Build history of the part. All positions in model axes, mm. Face numbers are marked on the shaded views. Give positions to 0.01 mm unless a question says otherwise; leave off trailing zeros. Order: outer loops, then holes, each group sorted by start corner. A loop starts at its lowest first (then second) coordinate and runs counter-clockwise, first axis right, second up. Notation, with made-up numbers: (33, -7.75) -> (44, -7.75) arc R15 cw to (44, 16.25) -> close; hole circle Ø1 at (-25.5, 61.25). An arc over 180 degrees is marked (long way). Write item = value, one per line. Start each with the question number.
from build123d import *

# Parameters (mm, degrees)
SKETCH_1_W          = 8
SKETCH_1_H          = 5
SKETCH_1_R          = 1.949999999
SKETCH_1_R_2        = 4
SKETCH_1_R_3        = 2
BOSS_EXTRUDE1_DEPTH = 10


with BuildPart() as part:
    # Sketch 1 → Boss-Extrude1 (new body)
    with BuildSketch(Plane.XY):
        with BuildLine():
            ThreePointArc((27.5, 18), (33.863961031, 15.363961031), (36.5, 9))
            Line((36.5, 9), (36.5, 41))
            Line((36.5, 41), (-6.9, 41))
            ThreePointArc((-6.9, 41), (-1.243145751, 38.656854249), (1.1, 33))
            Line((1.1, 33), (1.1, 28))
            ThreePointArc((1.1, 28), (4.028932188, 20.928932188), (11.1, 18))
            Line((11.1, 18), (27.5, 18))
        make_face()
        with BuildLine():
            ThreePointArc((-27.5, 12), (-33.5, 6), (-27.5, 0))
            Line((-27.5, 0), (27.5, 0))
            ThreePointArc((27.5, 0), (33.863961031, 2.636038969), (36.5, 9))
            ThreePointArc((36.5, 9), (33.863961031, 15.363961031), (27.5, 18))
            Line((27.5, 18), (11.1, 18))
            ThreePointArc((11.1, 18), (4.028932188, 20.928932188), (1.1, 28))
            Line((1.1, 28), (1.1, 33))
            ThreePointArc((1.1, 33), (-1.243145751, 38.656854249), (-6.9, 41))
            ThreePointArc((-6.9, 41), (-12.556854249, 38.656854249), (-14.9, 33))
            Line((-14.9, 33), (-14.9, 22))
            ThreePointArc((-14.9, 22), (-17.828932188, 14.928932188), (-24.9, 12))
            Line((-24.9, 12), (-27.5, 12))
        make_face()
        with Locations((-11.5, 6)):
            Rectangle(SKETCH_1_W, SKETCH_1_H, mode=Mode.SUBTRACT)
        with Locations((-1.238171752, 11.18329463)):
            Circle(SKETCH_1_R, mode=Mode.SUBTRACT)
        with Locations((6.5, 6)):
            Rectangle(SKETCH_1_W, SKETCH_1_H, mode=Mode.SUBTRACT)
        with Locations((27.5, 9)):
            Circle(SKETCH_1_R_2, mode=Mode.SUBTRACT)
        with Locations((-6.9, 33)):
            Circle(SKETCH_1_R_3, mode=Mode.SUBTRACT)
    extrude(amount=BOSS_EXTRUDE1_DEPTH)


solid = part.part
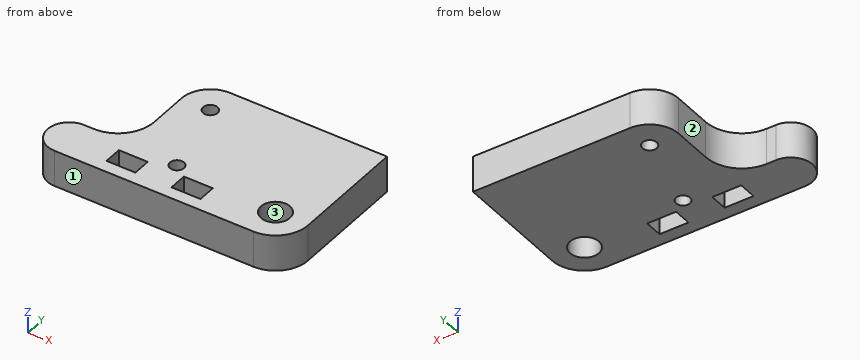
(1) Wall check: line 1 (X direction, y = 4, z = 7.25); line 2 (Y direction, x = -6.9, z = 2.75); line 3 (X direction, y = 28, z = 7.75). Give the ranges that are in metal, low to high. Write a range as [from, to].
(2) Mould opens along X. For the marked faces 1, 2 and 3 say: released by +X, released by -X, zero draft, split by the parting line, or undercut.
(3) Flat gauge pins, fed straight in: P1, Ø2, axis at x = -25.5, z = 4.5, coming from the +Y side; P2, Ø2.5, axis at y = 5.5, z = 4, coming from the +X side; P3, Ø1.5, axis at y = 6.5, z = 4.5, coming from the +X side. Where does each tip first touch, or does it go through?
(4) Cut at B-B, the plane y = 6. Give the cut face in (x, z), plus the area to 3 significant figures.
(5) Cut at D-D, the plane x = 24.5. Give the cut face in (y, z).
(6) Cut at A-A, the plane x = 4.5. Give the cut face in (y, z), plus the area to 3 significant figures.
(7) Cut at C-C, the plane z = 7. Give the cut face in (x, y), plus the area to 3 significant figures.
Results:
q1.line_1 = [-33.16, -15.5], [-7.5, 2.5], [10.5, 34.98]
q1.line_2 = [0, 31], [35, 41]
q1.line_3 = [-14.9, 36.5]
q2.face_1 = zero draft
q2.face_2 = released by -X
q2.face_3 = undercut
q3.P1 = 12.01
q3.P2 = 36.21
q3.P3 = 36.33
q4.outline = (-33.5, 0) -> (-15.5, 0) -> (-15.5, 10) -> (-33.5, 10) -> close; (-7.5, 0) -> (2.5, 0) -> (2.5, 10) -> (-7.5, 10) -> close; (10.5, 0) -> (24.85, 0) -> (24.85, 10) -> (10.5, 10) -> close; (30.15, 0) -> (35.99, 0) -> (35.99, 10) -> (30.15, 10) -> close
q4.area = 482 mm2
q5.outline = (0, 0) -> (6.35, 0) -> (6.35, 10) -> (0, 10) -> close; (11.65, 0) -> (41, 0) -> (41, 10) -> (11.65, 10) -> close
q6.outline = (0, 0) -> (3.5, 0) -> (3.5, 10) -> (0, 10) -> close; (8.5, 0) -> (41, 0) -> (41, 10) -> (8.5, 10) -> close
q6.area = 360 mm2
q7.outline = (-27.5, 0) -> (27.5, 0) arc R9 ccw to (36.5, 9) -> (36.5, 41) -> (-6.9, 41) arc R8 ccw to (-14.9, 33) -> (-14.9, 22) arc R10 cw to (-24.9, 12) -> (-27.5, 12) arc R6 ccw to start; hole (-15.5, 3.5) -> (-7.5, 3.5) -> (-7.5, 8.5) -> (-15.5, 8.5) -> close; hole circle Ø4 at (-6.9, 33); hole circle Ø3.9 at (-1.24, 11.18); hole (2.5, 3.5) -> (10.5, 3.5) -> (10.5, 8.5) -> (2.5, 8.5) -> close; hole circle Ø8 at (27.5, 9)
q7.area = 2,150 mm2
